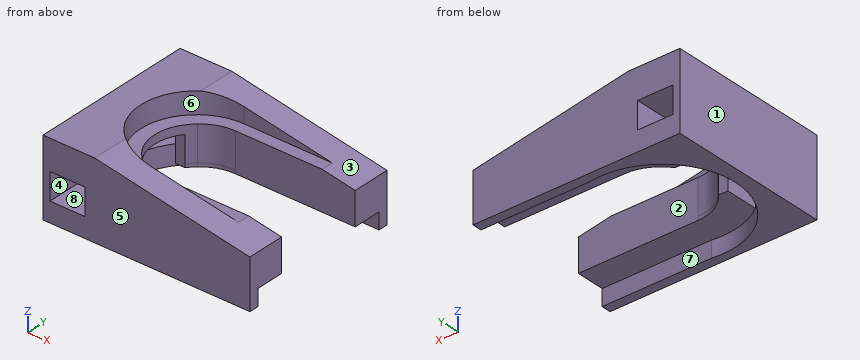
```python
from build123d import *

# Parameters (mm, degrees)
SKETCH_1_24X19_W         = 19
SKETCH_1_24X19_H         = 24
EXTRUDE_1_33_DEPTH       = 33
CUT_EXTRUDE_2_REACH      = 38.377
CUT_EXTRUDE_4_2_DEPTH    = 1.9
CUT_EXTRUDE_6_3_REACH    = 29.71
SKETCH_7_5_W             = 24
SKETCH_7_5_H             = 19
EXTRUDE_7_DEPTH          = 5
CUT_EXTRUDE_10_4_REACH   = 41.925
SKETCH_11_W              = 8.5
SKETCH_11_H              = 3.1
CUT_EXTRUDE_11_5_DEPTH   = 4.9
SKETCH_11D1_W            = 6
SKETCH_11D1_H            = 3.1
CUT_EXTRUDE_11D1_6_DEPTH = 10
CUT_EXTRUDE_12_9_REACH   = 31.655
CUT_EXTRUDE_11_DEPTH     = 3.5
SKETCH_5903_W            = 53.98
SKETCH_5903_H            = 19
CUT_EXTRUDE_12_DEPTH     = 1
CUT_EXTRUDE_13_DEPTH     = 40.102429623
CUT_EXTRUDE_15_REACH     = 33.036
SKETCH_5021_R            = 3.5
EXTRUDE_2_DEPTH          = 0.4
SKETCH_7445_W            = 0.8
SKETCH_7445_H            = 3.1
EXTRUDE_3_DEPTH          = 19
CUT_EXTRUDE_16_DEPTH     = 32.036269144
SKETCH_14_W              = 54.018014823
SKETCH_14_H              = 29.926878018
CUT_EXTRUDE_17_DEPTH     = 28.710286942


with BuildPart() as part:
    # 1底部方形_24x19 → 1凸台-拉伸_高33 (new body)
    with BuildSketch(Plane(origin=(0, 0, 0), x_dir=(0, 1, 0), z_dir=(0, 0, 1))):
        Rectangle(SKETCH_1_24X19_W, SKETCH_1_24X19_H)
    extrude(amount=EXTRUDE_1_33_DEPTH)

    # 2吸嘴停靠渐变槽 → 2切除-拉伸 (cut, up to next)
    with BuildSketch(Plane.XY.offset(33), mode=Mode.PRIVATE) as cut_extrude_2_sk1:
        with BuildLine():
            Line((12, -5.1), (12, 5.1))
            Line((12, 5.1), (-1.9, 5.1))
            add(Edge.make_bspline(
                [(-5.213938048, 3.830222216), (-3.829124073, 5.093205317), (-1.9, 5.1)],
                knots=[0, 0, 0, 1, 1, 1], degree=2))
            ThreePointArc((-5.213938048, 3.830222216), (-7, 0), (-5.213938048, -3.830222216))
            add(Edge.make_bspline(
                [(-5.213938048, -3.830222216), (-3.829124073, -5.093205317), (-1.9, -5.1)],
                knots=[0, 0, 0, 1, 1, 1], degree=2))
            Line((-1.9, -5.1), (12, -5.1))
        make_face()
    cut_extrude_2_tool1 = extrude(cut_extrude_2_sk1.sketch, amount=-CUT_EXTRUDE_2_REACH, mode=Mode.PRIVATE) & part.part
    add(cut_extrude_2_tool1.solids().sort_by_distance((3.017719, 0, 33))[0], mode=Mode.SUBTRACT)

    # 4反光板停靠槽 → 4切除-拉伸2 (cut)
    with BuildSketch(Plane.XY.offset(25)):
        with BuildLine():
            Line((-0.7, 8.4), (12, 8.4))
            Line((12, 8.4), (12, -8.4))
            Line((12, -8.4), (-0.7, -8.4))
            ThreePointArc((-0.7, -8.4), (-10.5, 0), (-0.7, 8.4))
        make_face()
    extrude(amount=-CUT_EXTRUDE_4_2_DEPTH, mode=Mode.SUBTRACT)

    # 6反光板小圆柱 → 6切除-拉伸3 (cut, up to next)
    with BuildSketch(Plane.XY.offset(23.1), mode=Mode.PRIVATE) as cut_extrude_6_3_sk1:
        with BuildLine():
            Line((-2.1, -6.3), (12, -6.3))
            Line((12, -6.3), (12, 6.3))
            Line((12, 6.3), (-2.1, 6.3))
            ThreePointArc((-2.1, 6.3), (-8.4, 0), (-2.1, -6.3))
        make_face()
    cut_extrude_6_3_tool1 = extrude(cut_extrude_6_3_sk1.sketch, amount=-CUT_EXTRUDE_6_3_REACH, mode=Mode.PRIVATE) & part.part
    add(cut_extrude_6_3_tool1.solids().sort_by_distance((2.424095, 0, 23.1))[0], mode=Mode.SUBTRACT)

    # 7草图5 → 7凸台-拉伸_底板厚度 (add)
    with BuildSketch(Plane(origin=(0, 0, 0), x_dir=(1, 0, 0), z_dir=(0, 0, -1))):
        Rectangle(SKETCH_7_5_W, SKETCH_7_5_H)
    extrude(amount=-EXTRUDE_7_DEPTH)

    # 10切除-拉伸4: up to this face of the body (flat: up to its plane)
    cut_extrude_10_4_end = Plane(part.part.faces().sort_by_distance((0, -9.5, 16.5))[0])
    # Sketch 10 → 10切除-拉伸4 (cut, up to the picked face)
    with BuildSketch(Plane(origin=(0, 9.5, 0), x_dir=(-1, 0, 0), z_dir=(0, 1, 0)), mode=Mode.PRIVATE) as cut_extrude_10_4_sk1:
        Polygon((-12, 31.162738066), (-12, 33), (9, 33), align=None)
    cut_extrude_10_4_tool1 = split(extrude(cut_extrude_10_4_sk1.sketch, amount=-CUT_EXTRUDE_10_4_REACH, mode=Mode.PRIVATE), bisect_by=cut_extrude_10_4_end, keep=Keep.BOTH, mode=Mode.PRIVATE)
    add(cut_extrude_10_4_tool1.solids().sort_by(Axis((5, 9.5, 32.387579), (0, -1, 0)))[0], mode=Mode.SUBTRACT)

    # Sketch 11 → 11切除-拉伸5 (cut)
    with BuildSketch(Plane(origin=(-12, 0, 0), x_dir=(0, -1, 0), z_dir=(-1, 0, 0))):
        with Locations((-5.25, 26.95)):
            Rectangle(SKETCH_11_W, SKETCH_11_H)
        with Locations((5.25, 26.95)):
            Rectangle(SKETCH_11_W, SKETCH_11_H)
    extrude(amount=-CUT_EXTRUDE_11_5_DEPTH, mode=Mode.SUBTRACT)

    # 11d1_磁铁开窗 → 11d1切除-拉伸6 (cut)
    with BuildSketch(Plane(origin=(-12, 0, 0), x_dir=(0, -1, 0), z_dir=(-1, 0, 0))):
        with Locations((0, 26.95)):
            Rectangle(SKETCH_11D1_W, SKETCH_11D1_H)
    extrude(amount=-CUT_EXTRUDE_11D1_6_DEPTH, mode=Mode.SUBTRACT)

    # 12切除薄壁 → 12切除-拉伸9 (cut, up to next)
    with BuildSketch(Plane.XY.offset(25.4), mode=Mode.PRIVATE) as cut_extrude_12_9_sk1:
        with BuildLine():
            Line((-0.7, 8.4), (-0.7, -8.4))
            ThreePointArc((-0.7, -8.4), (-10.5, 0), (-0.7, 8.4))
        make_face()
    cut_extrude_12_9_tool1 = extrude(cut_extrude_12_9_sk1.sketch, amount=-CUT_EXTRUDE_12_9_REACH, mode=Mode.PRIVATE) & part.part
    add(cut_extrude_12_9_tool1.solids().sort_by_distance((-4.916056, 0, 25.4))[0], mode=Mode.SUBTRACT)

    # Sketch 5393 → 切除-拉伸11 (cut)
    with BuildSketch(Plane.XY.offset(33)):
        with BuildLine():
            Line((-2.099999748, 6.5), (12, 6.5))
            Line((12, 6.5), (12, -6.5))
            Line((12, -6.5), (-2.099999748, -6.5))
            ThreePointArc((-2.099999748, -6.5), (-8.6, 0), (-2.099999748, 6.5))
        make_face()
    extrude(amount=-CUT_EXTRUDE_11_DEPTH, mode=Mode.SUBTRACT)

    # Sketch 5903 → 切除-拉伸12 (cut)
    with BuildSketch(Plane.XY.offset(33)):
        with Locations((14.99, 0)):
            Rectangle(SKETCH_5903_W, SKETCH_5903_H)
    extrude(amount=-CUT_EXTRUDE_12_DEPTH, mode=Mode.SUBTRACT)

    # Sketch 6208 → 切除-拉伸13 (cut, through all)
    with BuildSketch(Plane.XZ.offset(9.5)):
        Polygon((2.430052303, 32), (12, 31.162738066), (12, 28.826114347), (-6, 32), align=None)
    extrude(amount=-CUT_EXTRUDE_13_DEPTH, mode=Mode.SUBTRACT)

    # Sketch 5021 → 切除-拉伸15 (cut, up to next)
    with BuildSketch(Plane.XY.offset(5), mode=Mode.PRIVATE) as cut_extrude_15_sk1:
        with Locations((2, 0)):
            Circle(SKETCH_5021_R)
    cut_extrude_15_tool1 = extrude(cut_extrude_15_sk1.sketch, amount=-CUT_EXTRUDE_15_REACH, mode=Mode.PRIVATE) & part.part
    add(cut_extrude_15_tool1.solids().sort_by_distance((2, 0, 5))[0], mode=Mode.SUBTRACT)

    # Sketch 6983 → 凸台-拉伸2 (add)
    with BuildSketch(Plane(origin=(0, 0, 25.4), x_dir=(1, 0, 0), z_dir=(0, 0, -1))):
        with BuildLine():
            Line((-7.1, -3), (-7.1, -6.8))
            ThreePointArc((-7.1, -6.8), (-4.061552813, -8.246211251), (-0.7, -8.4))
            Line((-0.7, -8.4), (-0.7, -5.1))
            Line((-0.7, -5.1), (-1.9, -5.1))
            add(Edge.make_bspline(
                [(-1.9, -5.1), (-3.829124073, -5.093205317), (-5.213938048, -3.830222216)],
                knots=[0, 0, 0, 1, 1, 1], degree=2))
            ThreePointArc((-5.213938048, -3.830222216), (-5.630777158, -3.437652866), (-6, -3))
            Line((-6, -3), (-7.1, -3))
        make_face()
        with BuildLine():
            Line((-7.1, 3), (-6, 3))
            ThreePointArc((-6, 3), (-5.630777158, 3.437652866), (-5.213938048, 3.830222216))
            add(Edge.make_bspline(
                [(-5.213938048, 3.830222216), (-3.829124073, 5.093205317), (-1.9, 5.1)],
                knots=[0, 0, 0, 1, 1, 1], degree=2))
            Line((-1.9, 5.1), (-0.7, 5.1))
            Line((-0.7, 5.1), (-0.7, 8.4))
            ThreePointArc((-0.7, 8.4), (-4.061552813, 8.246211251), (-7.1, 6.8))
            Line((-7.1, 6.8), (-7.1, 3))
        make_face()
    extrude(amount=EXTRUDE_2_DEPTH)

    # Sketch 7445 → 凸台-拉伸3 (add)
    with BuildSketch(Plane.XZ.offset(9.5)):
        with Locations((-11.6, 26.95)):
            Rectangle(SKETCH_7445_W, SKETCH_7445_H)
    extrude(amount=-EXTRUDE_3_DEPTH)

    # 草图13 → 切除-拉伸16 (cut, through all)
    with BuildSketch(Plane.XY.offset(5)):
        with BuildLine():
            Line((-2.1, -6.3), (12, -6.3))
            Line((12, -6.3), (12, 6.3))
            Line((12, 6.3), (-2.1, 6.3))
            ThreePointArc((-2.1, 6.3), (-8.4, 0), (-2.1, -6.3))
        make_face()
    extrude(amount=-CUT_EXTRUDE_16_DEPTH, mode=Mode.SUBTRACT)

    # 草图14 → 切除-拉伸17 (cut, through all)
    with BuildSketch(Plane.XY.offset(23.1)):
        with Locations((6.444750957, 0.291135192)):
            Rectangle(SKETCH_14_W, SKETCH_14_H)
    extrude(amount=-CUT_EXTRUDE_17_DEPTH, mode=Mode.SUBTRACT)


solid = part.part
```
Can you work these out from the model? Positions are in its coordinate system, mm. Face numbers are marked on the shaded views. A direction names the side the tool comes from. Give positions to 0.01 mm unless a question says otherwise; leave off trailing zeros. Write each loop counter-clockwise with the first axis right and the second up, starting at its lowest first coordinate (ties: lowest second). Pieces come first, ordered by that corner, then holes. Notation, with made-up numbers: (42, 31.25) -> (76, 31.25) arc R13 ccw to (76, 46.25) -> close; hole circle Ø11 at (-23.75, 11.25). An arc over 180 degrees is marked (long way). One line per item, written item: value.
Q1. Imagine slicing it at A-A on y = -7.5. Please give me the cut outline in (x, z).
Results found:
outline: (-12, 23.1) -> (-6, 23.1) -> (-6, 25) -> (12, 25) -> (12, 28.83) -> (-6, 32) -> (-12, 32) -> close; hole (-11.2, 25.4) -> (-7.1, 25.4) -> (-7.1, 28.5) -> (-11.2, 28.5) -> close
Q2. Imagine slicing it at B-B on y = 0. Please give me the cut outline in (x, z), and give its area (3 significant figures).
Results found:
outline: (-12, 23.1) -> (-10.5, 23.1) -> (-10.5, 25.4) -> (-11.2, 25.4) -> (-11.2, 28.5) -> (-7, 28.5) -> (-7, 29.5) -> (-8.6, 29.5) -> (-8.6, 32) -> (-12, 32) -> close
area: 19.4 mm^2
Q3. Imagine slicing it at C-C on x = 8.75. Please give me the cut outline in (y, z), and give its area (3 significant figures).
Results found:
outline: (-9.5, 23.1) -> (-8.4, 23.1) -> (-8.4, 25) -> (-5.1, 25) -> (-5.1, 29.4) -> (-9.5, 29.4) -> close; (5.1, 25) -> (8.4, 25) -> (8.4, 23.1) -> (9.5, 23.1) -> (9.5, 29.4) -> (5.1, 29.4) -> close
area: 42.9 mm^2
Q4. Which directions (+Z, -Z, +X, -X, +Y, -Y) give clear straight access to the entire face, cutting with the end or side of a thin tool? Please do the marked faces 5, 6, 7 and 8.
Results found:
face 5: +Z, -Z, +X, -X, -Y
face 6: +Z, +X
face 7: -Z, +X
face 8: +Y, -Y
Q5. We'd pull the mould along X, two halves only. Please class the marked faces 1, 2, 3 and 4: +X half, -X half, draft (parallel to the pull), parting line (faces both ways), or undercut.
Results found:
face 1: -X half
face 2: draft
face 3: +X half
face 4: undercut
Q6. Please list where these lines run through material, in increasing order: line 1 (Y direction, x = -2, z = 24.6); line 2 (Y direction, x = -1, z = 30.75); line 3 (Z direction, x = -11, y = 3.5). Write a range as [from, to].
Results found:
line 1: y = [-9.5, -8.5], [8.5, 9.5]
line 2: y = [-9.5, -6.5], [6.5, 9.5]
line 3: z = [23.1, 25.4], [28.5, 32]
Q7. For P1, Ø0.5, axis at x = 2, z = 31, coming from the +Y side; P2, Ø6, axis at x = -1, y = 2.5, coming from the +Z side, each with a flat end and sliding along its axis, tell me the tip position at first contact or that it passes through.
Results found:
P1: passes through
P2: stops at z = 29.5
Q8. Imagine slicing it at D-D on z = 28. Give the number of separate pieces and of enclosed holes in the cut face, and give its area (3 significant figures).
Results found:
separate pieces: 3
enclosed holes: 0
area: 193 mm^2
